The model under review builds one solid part; all positions refer to its coordinate system, in mm. Face numbers are marked on the shaded views. A direction names the side the tool comes from. Round coordinates to 2 decimals unless told otherwise and drop trailing zeros. Loops run counter-clockwise (first coordinate to the right, second up) from the corner with the lowest first, then second, coordinate; pieces in that order, holes last. Notation, with made-up numbers: M -6,19.5 L 16,19.5 A27 cw 16,37.5 Z; hole C 22.5,38.5 d10. An arc over 180 degrees is marked long. Use a Markdown table: item, result. Add a question column.
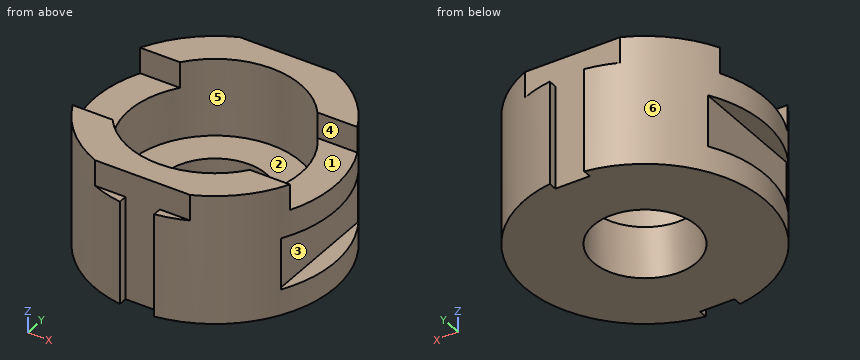
```python
from build123d import *

# Parameters (mm, degrees)
SKETCH1_R           = 70
BOSS_EXTRUDE1_DEPTH = 75
SKETCH2_R           = 30
CUT_EXTRUDE1_DEPTH  = 75
CUT_EXTRUDE2_DEPTH  = 75
CUT_EXTRUDE3_DEPTH  = 75
SKETCH5_W           = 30
SKETCH5_H           = 70
CUT_EXTRUDE5_DEPTH  = 75
SKETCH6_W           = 30
SKETCH6_H           = 70
CUT_EXTRUDE6_DEPTH  = 75
SKETCH7_W           = 50
SKETCH7_H           = 15
CUT_EXTRUDE11_DEPTH = 5
CUT_EXTRUDE12_DEPTH = 88
SKETCH12_W          = 15
SKETCH12_H          = 1.10145185
CUT_EXTRUDE14_DEPTH = 88
SKETCH13_W          = 15
SKETCH13_H          = 1.10145185
CUT_EXTRUDE15_DEPTH = 88
SKETCH14_W          = 50
SKETCH14_H          = 15
CUT_EXTRUDE16_DEPTH = 5
SKETCH15_W          = 20
SKETCH15_H          = 5
CUT_EXTRUDE17_DEPTH = 73
SKETCH16_W          = 15
SKETCH16_H          = 1.10145185
CUT_EXTRUDE18_DEPTH = 73
SKETCH17_W          = 15
SKETCH17_H          = 1.10145185
CUT_EXTRUDE19_DEPTH = 73
CUT_EXTRUDE20_DEPTH = 15
SKETCH20_R          = 50
CUT_EXTRUDE21_DEPTH = 45


with BuildPart() as part:
    # Sketch1 → Boss-Extrude1 (new body)
    with BuildSketch(Plane.XY):
        Circle(SKETCH1_R)
    extrude(amount=BOSS_EXTRUDE1_DEPTH)

    # Sketch2 → Cut-Extrude1 (cut)
    with BuildSketch(Plane.XY.offset(75)):
        Circle(SKETCH2_R)
    extrude(amount=-CUT_EXTRUDE1_DEPTH, mode=Mode.SUBTRACT)

    # Sketch3 → Cut-Extrude2 (cut)
    with BuildSketch(Plane.XY.offset(75)):
        with BuildLine():
            Line((-10, 69.282032303), (10, 69.282032303))
            ThreePointArc((10, 69.282032303), (0, 70), (-10, 69.282032303))
        make_face()
    extrude(amount=-CUT_EXTRUDE2_DEPTH, mode=Mode.SUBTRACT)

    # Sketch4 → Cut-Extrude3 (cut)
    with BuildSketch(Plane.XY.offset(75)):
        with BuildLine():
            ThreePointArc((-10, -69.282032303), (0, -70), (10, -69.282032303))
            Line((10, -69.282032303), (-10, -69.282032303))
        make_face()
    extrude(amount=-CUT_EXTRUDE3_DEPTH, mode=Mode.SUBTRACT)

    # Sketch5 → Cut-Extrude5 (cut)
    with BuildSketch(Plane(origin=(-60, 0, 0), x_dir=(0, 0, -1), z_dir=(1, 0, 0))):
        with Locations((-30, 0.717967697)):
            Rectangle(SKETCH5_W, SKETCH5_H)
    extrude(amount=-CUT_EXTRUDE5_DEPTH, mode=Mode.SUBTRACT)

    # Sketch6 → Cut-Extrude6 (cut)
    with BuildSketch(Plane(origin=(60, 0, 0), x_dir=(0, 0, -1), z_dir=(1, 0, 0))):
        with Locations((-30, 0.717967697)):
            Rectangle(SKETCH6_W, SKETCH6_H)
    extrude(amount=CUT_EXTRUDE6_DEPTH, mode=Mode.SUBTRACT)

    # Sketch7 → Cut-Extrude11 (cut)
    with BuildSketch(Plane(origin=(0, 69.282032303, 0), x_dir=(1, 0, 0), z_dir=(0, 1, 0))):
        with Locations((0, -67.5)):
            Rectangle(SKETCH7_W, SKETCH7_H)
    extrude(amount=-CUT_EXTRUDE11_DEPTH, mode=Mode.SUBTRACT)

    # Sketch10 → Cut-Extrude12 (cut)
    with BuildSketch(Plane.XY.offset(60)):
        Polygon((-10, 69.282032303), (-10, 64.282032303), (10.07167941, 64.282032303), (10, 69.282032303), align=None)
    extrude(amount=-CUT_EXTRUDE12_DEPTH, mode=Mode.SUBTRACT)

    # Sketch12 → Cut-Extrude14 (cut)
    with BuildSketch(Plane(origin=(-25, 0, 0), x_dir=(0, 0, -1), z_dir=(1, 0, 0))):
        with Locations((-67.5, 64.832758228)):
            Rectangle(SKETCH12_W, SKETCH12_H)
    extrude(amount=-CUT_EXTRUDE14_DEPTH, mode=Mode.SUBTRACT)

    # Sketch13 → Cut-Extrude15 (cut)
    with BuildSketch(Plane.ZY.offset(-25)):
        with Locations((67.5, 64.832758228)):
            Rectangle(SKETCH13_W, SKETCH13_H)
    extrude(amount=-CUT_EXTRUDE15_DEPTH, mode=Mode.SUBTRACT)

    # Sketch14 → Cut-Extrude16 (cut)
    with BuildSketch(Plane.XZ.offset(69.282032303)):
        with Locations((0, 67.5)):
            Rectangle(SKETCH14_W, SKETCH14_H)
    extrude(amount=-CUT_EXTRUDE16_DEPTH, mode=Mode.SUBTRACT)

    # Sketch15 → Cut-Extrude17 (cut)
    with BuildSketch(Plane.XY.offset(60)):
        with Locations((0, -66.782032303)):
            Rectangle(SKETCH15_W, SKETCH15_H)
    extrude(amount=-CUT_EXTRUDE17_DEPTH, mode=Mode.SUBTRACT)

    # Sketch16 → Cut-Extrude18 (cut)
    with BuildSketch(Plane.ZY.offset(-25)):
        with Locations((67.5, -64.832758228)):
            Rectangle(SKETCH16_W, SKETCH16_H)
    extrude(amount=-CUT_EXTRUDE18_DEPTH, mode=Mode.SUBTRACT)

    # Sketch17 → Cut-Extrude19 (cut)
    with BuildSketch(Plane(origin=(-25, 0, 0), x_dir=(0, 0, -1), z_dir=(1, 0, 0))):
        with Locations((-67.5, -64.832758228)):
            Rectangle(SKETCH17_W, SKETCH17_H)
    extrude(amount=-CUT_EXTRUDE19_DEPTH, mode=Mode.SUBTRACT)

    # Sketch18 → Cut-Extrude20 (cut)
    with BuildSketch(Plane.XY.offset(75)):
        with BuildLine():
            ThreePointArc((0, -30), (-30, 0), (0, 30))
            Line((0, 30), (-63.245553203, 30))
            ThreePointArc((-63.245553203, 30), (-70, 0), (-63.245553203, -30))
            Line((-63.245553203, -30), (0, -30))
        make_face()
        with BuildLine():
            Line((63.245553203, 30), (0, 30))
            ThreePointArc((0, 30), (21.213203436, 21.213203436), (30, 0))
            ThreePointArc((30, 0), (21.213203436, -21.213203436), (0, -30))
            Line((0, -30), (63.245553203, -30))
            ThreePointArc((63.245553203, -30), (70, 0), (63.245553203, 30))
        make_face()
    extrude(amount=-CUT_EXTRUDE20_DEPTH, mode=Mode.SUBTRACT)

    # Sketch20 → Cut-Extrude21 (cut)
    with BuildSketch(Plane.XY.offset(75)):
        Circle(SKETCH20_R)
    extrude(amount=-CUT_EXTRUDE21_DEPTH, mode=Mode.SUBTRACT)


solid = part.part
```
(1) Draft analysis for pull direction X (two halves, no side actions). For the marked faces 4, 5 and 6, state which applies: released by +X, released by -X, zero draft, split by the parting line, or undercut.
(2) Consider section C-C, the plane z = 5.5. Give the boundary of the cut face in (x, y), then the cut area to 3 significant figures.
(3) For the marked faces 1, 2 and 3, list the 3-axis set-ups (+Z, -Z, +X, -X, +Y, -Y) from which the entire face can be reached by the end or side of a thin tool; tool diameter is ignored.
(4) Insertion check: pin 1 Ø5 at (x, y) = (-66, -14) entering from -Z; pin 2 Ø6 at (y, z) = (7, 54.5) entering from +X; pin 3 Ø1.5 at (y, z) = (19, 55.5) entering from -X; pin 4 Ø2 at (x, z) = (-12, 23) entering from -Y. Each pin has a flat end and moves straight along its axis. Give the tip position at first contact, or say it passes through.
(5) Consider section A-A, the plane y = 0. Give the boundary of the cut face in (x, z).
(6) Consider section D-D, the plane z = 55. Give the boundary of the cut face in (x, y), then the cut area to 3 significant figures.
(7) Consider section B-B, the plane x = 0. Give the boundary of the cut face in (y, z), then the cut area to 3 significant figures.
(8) To check wall thickness, follow probe 1 along Y at (x, z) = (0, 47); probe 2 along Y at (x, z) = (0, 20); probe 3 along X at (y, z) = (0, 43). State the ranges of each line that lie inside material, in increasing order.
Found:
| question | item | result |
|---|---|---|
| 1 | face 4 | zero draft |
| 1 | face 5 | undercut |
| 1 | face 6 | released by -X |
| 2 | outline | M -10,-69.28 L -10,-64.28 L 10,-64.28 L 10,-69.28 A70 ccw 10,69.28 L 10.07,64.28 L -10,64.28 L -10,69.28 A70 ccw Z; hole C 0,0 d60 |
| 2 | area | 12,300 mm^2 |
| 3 | face 1 | +Z, +X, -X |
| 3 | face 2 | +Z |
| 3 | face 3 | +X |
| 4 | pin 1 | stops at z = 0 |
| 4 | pin 2 | stops at x = 69.89 |
| 4 | pin 3 | stops at x = -67.58 |
| 4 | pin 4 | stops at y = -69.13 |
| 5 | outline | M -70,0 L -30,0 L -30,30 L -50,30 L -50,60 L -70,60 L -70,45 L -60,45 L -60,15 L -70,15 Z; M 30,0 L 70,0 L 70,15 L 60,15 L 60,45 L 70,45 L 70,60 L 50,60 L 50,30 L 30,30 Z |
| 6 | outline | M -10,-69.28 L -10,-64.28 L 10,-64.28 L 10,-69.28 A70 ccw 10,69.28 L 10.07,64.28 L -10,64.28 L -10,69.28 A70 ccw Z; hole C 0,0 d100 |
| 6 | area | 7,320 mm^2 |
| 7 | outline | M -64.28,0 L -30,0 L -30,30 L -50,30 L -50,75 L -64.28,75 Z; M 30,0 L 64.28,0 L 64.28,75 L 50,75 L 50,30 L 30,30 Z |
| 7 | area | 3,340 mm^2 |
| 8 | probe 1 | y = -64.28 to -50, 50 to 64.28 |
| 8 | probe 2 | y = -64.28 to -30, 30 to 64.28 |
| 8 | probe 3 | x = -60 to -50, 50 to 60 |
